Can you work these out from the model? Positions are in its coordinate system, mm. A direction names the side the tool comes from. Give positions to 0.01 mm unless a question says otherwise; leave off trailing zeros. Loops run counter-clockwise (first coordinate to the right, second up) from the corner with the lowest first, then second, coordinate; pieces in that order, holes last. Notation, with made-up numbers: M 43.25,23 L 76.25,23 A33 cw 76.25,58 Z; hole C 41,8 d8. An arc over 180 degrees is marked long. Answer as a JSON object with one key per item and string values.
```python
from build123d import *

# Parameters (mm, degrees)
F0_W     = 21.45
F0_H     = 10.15
F1_DEPTH = 30.1
F2_W     = 4.5
F2_H     = 6
F2_W_2   = 5
F2_W_3   = 6
F3_DEPTH = 20
F4_W     = 6
F4_H     = 6
F5_DEPTH = 25
F6_W     = 38.292414
F6_H     = 55.741895
F7_DEPTH = 25


with BuildPart() as f1:
    # F0 (on Top) → F1 (new body)
    with BuildSketch(Plane.XY):
        Rectangle(F0_W, F0_H)
        Polygon((10.725, 7.226717), (10.725, 5.075), (10.725, -5.075), (13.978312, -5.075), (13.978312, 7.226717), align=None)
        Polygon((13.978312, 7.226717), (13.978312, -5.075), (17.385745, -5.075), (17.385745, 9.236451), (13.978312, 9.236451), align=None)
    extrude(amount=F1_DEPTH)

    # F2 (on face) → F3 (cut)
    with BuildSketch(Plane(origin=(-10.725, 0, 0), x_dir=(0, -1, 0), z_dir=(-1, 0, 0))):
        with Locations((-2.825, 6)):
            Rectangle(F2_W, F2_H)
        with Locations((-2.575, 15)):
            Rectangle(F2_W_2, F2_H)
        with Locations((-2.075, 24)):
            Rectangle(F2_W_3, F2_H)
    extrude(amount=-F3_DEPTH, mode=Mode.SUBTRACT)

    # F4 (on face) → F5 (cut)
    with BuildSketch(Plane.XZ.offset(5.075)):
        with Locations((-5.225, 6)):
            Rectangle(F4_W, F4_H)
        with Locations((-5.225, 15)):
            Rectangle(F4_W, F4_H)
        with Locations((-5.225, 24)):
            Rectangle(F4_W, F4_H)
    extrude(amount=-F5_DEPTH, mode=Mode.SUBTRACT)

    # F6 (on face) → F7 (cut)
    with BuildSketch(Plane.XZ.offset(5.075)):
        with Locations((19.921207, 9.509602)):
            Rectangle(F6_W, F6_H)
    extrude(amount=-F7_DEPTH, mode=Mode.SUBTRACT)


solid = f1.part
```
1) If we mould it in two halves opening along Z, with no side actions, what happens to faces 6 (the flat face through (-5, 0, 0)), 7 (the flat face through (-9, 0.075, 15)), 8 (the flat face through (-5, 5.075, 19)), 9 (the flat face through (-5, 0, 30.1))? For each: +Z half, -Z half, draft (parallel to the pull), parting line (faces both ways), or undercut.
Answer list:
{"face 6": "-Z half", "face 7": "undercut", "face 8": "draft", "face 9": "+Z half"}
2) Suppose I cut it at A-A, the plane y = -0.25. Write out the boundary of the cut face in (x, z) (3 decimals).
Answer list:
{"outline": "M -10.725,0 L 0.775,0 L 0.775,21 L -10.725,21 Z; M -10.725,27 L 0.775,27 L 0.775,30.1 L -10.725,30.1 Z; hole M -8.225,3 L -2.225,3 L -2.225,9 L -8.225,9 Z; hole M -8.225,12 L -2.225,12 L -2.225,18 L -8.225,18 Z"}
3) Suppose I cut it at D-D, the plane y = 1.5. Write out the boundary of the cut face in (x, z) (3 decimals), and give its area (3 significant figures).
Answer list:
{"outline": "M -10.725,0 L 0.775,0 L 0.775,3 L -10.725,3 Z; M -10.725,9 L 0.775,9 L 0.775,12 L -10.725,12 Z; M -10.725,18 L 0.775,18 L 0.775,21 L -10.725,21 Z; M -10.725,27 L 0.775,27 L 0.775,30.1 L -10.725,30.1 Z", "area": "139 mm^2"}
4) For faces 1 (the flat face through (-5, 5.075, 29)), 2 (the flat face through (-5, 1, 27)), 3 (the flat face through (-1, 0.075, 15)), 4 (the flat face through (-2.225, -3, 24)), 5 (the flat face through (0.775, -1, 15)), which set-ups out of +Z, -Z, +X, -X, +Y, -Y let a thin tool reach every point of the face, with its end or its side?
Answer list:
{"face 1": "+Z, -Z, +X, -X, +Y", "face 2": "+Y", "face 3": "+X, -X, +Y", "face 4": "+Y, -Y", "face 5": "+Z, -Z, +X, +Y, -Y"}
5) Please list where these lines run through material, in increasing order: line 1 along Z through (x, y) = (-5.5, -4.5); line 2 along X through (y, z) = (-3.5, 23) (3 decimals); line 3 along Z through (x, y) = (-1, -0.5). Write a range as from..to.
Answer list:
{"line 1": "0..3, 9..12, 18..21, 27..30.1", "line 2": "-10.725..-8.225, -2.225..0.775", "line 3": "0..21, 27..30.1"}
6) Suppose I cut it at C-C, the plane z = 23.5. Write out the boundary of the cut face in (x, y) (3 decimals), and give its area (3 significant figures).
Answer list:
{"outline": "M -10.725,-5.075 L -8.225,-5.075 L -8.225,-0.925 L -10.725,-0.925 Z; M -2.225,-5.075 L 0.775,-5.075 L 0.775,-0.925 L -2.225,-0.925 Z", "area": "22.8 mm^2"}
7) Will these pins go through, and if not, where does the flat tip stop? pin 1 Ø1.5 at (x, z) = (-1, 25) entering from +Y (3 decimals); pin 2 Ø3 at (x, z) = (-9.5, 6) entering from +Y (3 decimals); pin 3 Ø1.5 at (x, z) = (-6.5, 6) entering from +Y; pin 4 Ø3 at (x, z) = (-9, 15) entering from +Y (3 decimals).
Answer list:
{"pin 1": "y = -0.925", "pin 2": "y = 0.575", "pin 3": "through", "pin 4": "y = 0.075"}
8) Suppose I cut it at B-B, the plane x = -6. Write out the boundary of the cut face in (y, z) (3 decimals), and give its area (3 significant figures).
Answer list:
{"outline": "M -5.075,0 L 5.075,0 L 5.075,3 L -5.075,3 Z; M -5.075,9 L 5.075,9 L 5.075,12 L -5.075,12 Z; M -5.075,18 L 5.075,18 L 5.075,21 L -5.075,21 Z; M -5.075,27 L 5.075,27 L 5.075,30.1 L -5.075,30.1 Z", "area": "123 mm^2"}
